CAD build for the part. Positions are in the model's coordinates, mm. A direction names the side the tool comes from. Give positions to 0.01 mm unless a question says otherwise; leave off trailing zeros. Loops run counter-clockwise (first coordinate to the right, second up) from the corner with the lowest first, then second, coordinate; pieces in that order, holes last.
Item 1: Saw through at C-C on z = 54. Give the cut face in (x, y), plus the area to 3 significant figures.
Item 2: Probe probe 1 along Y at (x, z) = (46.5, 65); probe 2 along Y at (x, z) = (76.5, 67); probe 3 along Z at (x, y) = (50, 37). List the from-to ranges inside material, lowest first.
Item 3: Saw through at B-B on x = 50.8. Give the cut face in (y, z) (3 decimals), plus the area to 3 significant figures.
Item 4: Mould opens along X. For faces 1 (the cylindrical face through (42.224, 13.505, 34.436)), 2 (the cylindrical face through (125.485, 68.77, 34.436)), 3 (the flat face through (15, 20, 69.85)), 4 (the flat face through (99.953, 54.706, 34.436)) say: released by +X, released by -X, zero draft, split by the parting line, or undercut.
Item 5: Saw through at A-A on y = 8.5. Give the cut face in (x, z).
Item 6: Saw through at D-D on x = 81.5. Give the cut face in (y, z), plus the area to 3 significant figures.
Item 7: Which spindle directions (+Z, -Z, +X, -X, +Y, -Y) get a long thin tool onto all of the face, cutting with end or side? Do faces 5 (the cylindrical face through (71.086, -4.383, 74.317)), 6 (the flat face through (51, 41, 69.85)), 7 (the flat face through (51, -4, 75.692)). Say none if no direction does.
Item 8: Drop flat-ended pins along their axis: P1, Ø2.5, axis at y = -4.5, z = 65, coming from the +X side; P2, Ø10, axis at x = 81, y = 9, coming from the +Z side; P3, Ø3, axis at x = 48, y = 30.5, coming from the -Z side; P4, Ø1.5, axis at y = 40, z = 12, coming from the -X side. Give the stop position or say it passes through.
from build123d import *

# Parameters (mm, degrees)
F0_R      = 2.54
F1_DEPTH  = 69.85
F2_W      = 40.132
F2_H      = 38.862
F2_R      = 2.54
F2_H_2    = 4.318
F3_DEPTH  = 19.812
F4_SIZE   = 12.7
F6_DEPTH  = 8.89
F7_R      = 10.4775
F8_DEPTH  = 5.969
F9_R      = 12.7
F10_DEPTH = 2.54


with BuildPart() as f1:
    # F0 (on Top) → F1 (new body)
    with BuildSketch(Plane.XY):
        with BuildLine():
            Line((96.012, 38.862), (130.048, 38.862))
            Line((130.048, 38.862), (130.048, 57.5797104578))
            ThreePointArc((130.048, 57.5797104578), (125.3611227125, 68.8948331703), (114.046, 73.5817104578))
            Line((114.046, 73.5817104578), (108.2220946444, 73.5817104578))
            ThreePointArc((108.2220946444, 73.5817104578), (105.4062842868, 72.6117093515), (103.7852854611, 70.1132992724))
            Line((103.7852854611, 70.1132992724), (96.012, 38.862))
        make_face()
        with BuildLine():
            ThreePointArc((0, 4.572), (1.3391077964, 1.3391077964), (4.572, 0))
            Line((4.572, 0), (125.476, 0))
            ThreePointArc((125.476, 0), (128.7088922036, 1.3391077964), (130.048, 4.572))
            Line((130.048, 4.572), (130.048, 38.862))
            Line((130.048, 38.862), (96.012, 38.862))
            Line((96.012, 38.862), (4.572, 38.862))
            ThreePointArc((4.572, 38.862), (1.3391077964, 37.5228922036), (0, 34.29))
            Line((0, 34.29), (0, 4.572))
        make_face()
        with Locations((39.878, 14.478)):
            Circle(F0_R, mode=Mode.SUBTRACT)
    extrude(amount=F1_DEPTH)

    # F2 (on face) → F3 (join)
    with BuildSketch(Plane.XY.offset(69.85)):
        with Locations((50.8, 19.431)):
            Rectangle(F2_W, F2_H)
        with Locations((39.878, 14.478)):
            Circle(F2_R, mode=Mode.SUBTRACT)
        with Locations((50.8, 41.021)):
            Rectangle(F2_W, F2_H_2)
        with Locations((39.878, 14.478)):
            Circle(F2_R)
    extrude(amount=F3_DEPTH)

    # F4
    f4_edges = [f1.edges().sort_by_distance(p)[0] for p in [
        (70.866, 21.59, 89.662),
        (50.8, 43.18, 89.662),
        (30.734, 21.59, 89.662),
    ]]
    chamfer(f4_edges, length=F4_SIZE)

    # F5 (on Front) + F1_face1 (on face) → F6 (join)
    with BuildSketch(Plane.XZ):
        with BuildLine():
            ThreePointArc((29.21, 62.484), (30.5491077964, 59.2511077964), (33.782, 57.912))
            Line((33.782, 57.912), (67.818, 57.912))
            ThreePointArc((67.818, 57.912), (71.0508922036, 59.2511077964), (72.39, 62.484))
            Line((72.39, 62.484), (72.39, 71.12))
            ThreePointArc((72.39, 71.12), (71.0508922036, 74.3528922036), (67.818, 75.692))
            Line((67.818, 75.692), (33.782, 75.692))
            ThreePointArc((33.782, 75.692), (30.5491077964, 74.3528922036), (29.21, 71.12))
            Line((29.21, 71.12), (29.21, 62.484))
        make_face()
    with BuildSketch(Plane(origin=(50.292, 38.862, 34.925), x_dir=(-1, 0, 0), z_dir=(0, 1, 0))):
        Polygon((-45.72, 34.925), (-45.72, -34.925), (45.72, -34.925), (45.72, 34.925), (19.558, 34.925), (-20.574, 34.925), align=None)
    extrude(amount=F6_DEPTH, dir=(0, -1, 0))

    # F7 (on face) → F8 (join)
    with BuildSketch(Plane.XY.offset(69.85)):
        with Locations((85.598, 22.987)):
            Circle(F7_R)
    extrude(amount=F8_DEPTH)

    # F9 (on face) → F10 (cut)
    with BuildSketch(Plane(origin=(0, 38.862, 0), x_dir=(-1, 0, 0), z_dir=(0, 1, 0))):
        with Locations((-50.8, 34.925)):
            Circle(F9_R)
    extrude(amount=-F10_DEPTH, mode=Mode.SUBTRACT)


solid = f1.part
Results below:
1. outline: (0, 4.57) arc R4.57 ccw to (4.57, 0) - (125.48, 0) arc R4.57 ccw to (130.05, 4.57) - (130.05, 57.58) arc R16 ccw to (114.05, 73.58) - (108.22, 73.58) arc R4.57 ccw to (103.79, 70.11) - (96.01, 38.86) - (4.57, 38.86) arc R4.57 ccw to (0, 34.29) - close; hole circle Ø5.08 at (39.88, 14.48)
1. area: 5,990 mm2
2. probe 1: y = -8.89 to 38.86
2. probe 2: y = 0 to 38.86
2. probe 3: z = 0 to 22.25, 47.6 to 83.14
3. outline: (-8.89, 57.912) - (0, 57.912) - (0, 0) - (38.862, 0) - (38.862, 22.225) - (36.322, 22.225) - (36.322, 47.625) - (38.862, 47.625) - (38.862, 69.85) - (43.18, 69.85) - (43.18, 76.962) - (30.48, 89.662) - (0, 89.662) - (0, 75.692) - (-8.89, 75.692) - close
3. area: 3,580 mm2
4. face 1: undercut
4. face 2: released by +X
4. face 3: zero draft
4. face 4: released by -X
5. outline: (0, 0) - (130.05, 0) - (130.05, 69.85) - (70.87, 69.85) - (70.87, 76.96) - (58.17, 89.66) - (43.43, 89.66) - (30.73, 76.96) - (30.73, 69.85) - (0, 69.85) - close
6. outline: (0, 0) - (38.86, 0) - (38.86, 69.85) - (32.63, 69.85) - (32.63, 75.82) - (13.34, 75.82) - (13.34, 69.85) - (0, 69.85) - close
6. area: 2,830 mm2
7. face 5: +Z, +X, -Y
7. face 6: -Z, -X, +Y
7. face 7: +Z, +X, -X, -Y
8. P1: stops at x = 72.39
8. P2: stops at z = 75.82
8. P3: stops at z = 0
8. P4: stops at x = 96.11
